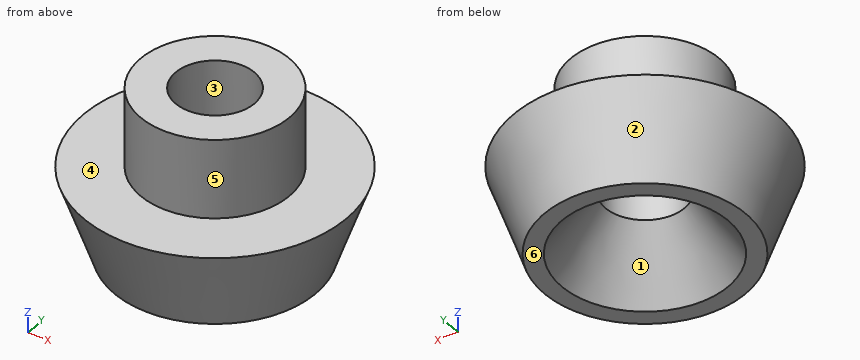
```python
from build123d import *

# Parameters (mm, degrees)
SKETCH_R         = 7.5
PAD_DEPTH        = 5
SKETCH001_R      = 4.25
PAD001_DEPTH     = 4.5
SKETCH002_R      = 2.25
POCKET_DEPTH     = 9.501
CHAMFER_SIZE2    = 3.5
CHAMFER_SIZE     = 2.5
CHAMFER001_SIZE2 = 4.999
CHAMFER001_SIZE  = 1.75


with BuildPart() as part:
    # Sketch → Pad (new body)
    with BuildSketch(Plane.XY):
        Circle(SKETCH_R)
    extrude(amount=PAD_DEPTH)

    # Sketch001 (on Face3 of Pad) → Pad001 (join)
    with BuildSketch(Plane.XY.offset(5)):
        Circle(SKETCH001_R)
    extrude(amount=PAD001_DEPTH)

    # Sketch002 (on Face5 of Pad001) → Pocket (cut, through all)
    with BuildSketch(Plane.XY.offset(9.5)):
        Circle(SKETCH002_R)
    extrude(amount=-POCKET_DEPTH, mode=Mode.SUBTRACT)

    # Chamfer
    chamfer_edges = [part.edges().sort_by_distance(p)[0] for p in [
        (-2.25, 0, 0),
    ]]
    chamfer_side = part.faces().sort_by_distance((-7.287868, 0, 0))[0]
    chamfer(chamfer_edges, length=CHAMFER_SIZE, length2=CHAMFER_SIZE2, reference=chamfer_side)

    # Chamfer001
    chamfer001_edges = [part.edges().sort_by_distance(p)[0] for p in [
        (-7.5, 0, 0),
    ]]
    chamfer001_side = part.faces().sort_by_distance((-4.962132, 0, 0))[0]
    chamfer(chamfer001_edges, length=CHAMFER001_SIZE, length2=CHAMFER001_SIZE2, reference=chamfer001_side)


solid = part.part
```
Source: CAD feature listing. Evaluate the final solid. Frame: model axes, mm. Face numbers are marked on the shaded views. A direction names the side the tool comes from. Give positions to 0.01 mm unless a question says otherwise; leave off trailing zeros. Write each loop counter-clockwise with the first axis right and the second up, starting at its lowest first coordinate (ties: lowest second). Pieces come first, ordered by that corner, then holes.
1. Material intervals for line 1 along Y through (x, z) = (0, 6.7); line 2 along Z through (x, y) = (5.5, -0.75); line 3 along Y through (x, z) = (0.25, 1.25), sorted ascending.
2. Access query for the marked faces 5 and 6. Directions: +Z, -Z, +X, -X, +Y, -Y. A direction counts if a zero-diameter tool reaches every point of the face in a straight line with its end or side. Return the directions, or none.
3. First-contact query: pin 1 (1.5 mm diameter, centred on x = 5.5, y = 4.5, fed in from +Z); pin 2 (3 mm diameter, centred on x = -5.5, z = 5, fed in from -Y); pin 3 (3 mm diameter, centred on x = -5, z = 4, fed in from +Y). Flat tips, straight axial feed; report the tip coordinate or a pass-through.
4. Section query D-D (z = 2.75). Return the cut outline in (x, y), then the cut area to 3 significant figures.
5. Section query C-C (z = 9). Return the cut outline in (x, y), then the cut area to 3 significant figures.
6. Pull-direction query (X, two-part tool) for the marked faces 1, 2, 3 and 4; classes: +X half, -X half, draft (parallel to the pull), parting line (faces both ways), or undercut.
Output values:
1. line 1: y = -4.25 to -2.25, 2.25 to 4.25
1. line 2: z = 0 to 5
1. line 3: y = -6.18 to -3.85, 3.85 to 6.18
2. face 5: +Z
2. face 6: -Z, +X, -X, +Y, -Y
3. pin 1: stops at z = 5
3. pin 2: stops at y = -6.34
3. pin 3: stops at y = 6.43
4. outline: circle Ø13.43 at (0, 0); hole circle Ø5.57 at (0, 0)
4. area: 117 mm2
5. outline: circle Ø8.5 at (0, 0); hole circle Ø4.5 at (0, 0)
5. area: 40.8 mm2
6. face 1: undercut
6. face 2: parting line
6. face 3: undercut
6. face 4: draft
